from build123d import *

# Parameters (mm, degrees)
SKETCH1_W                  = 50
SKETCH1_H                  = 15
SKETCH1_R                  = 2.025
BASE_FLANGE1_DEPTH         = 1
F_4_CLEARANCE_HOLE1_D      = 3.2639
SKETCHED_START             = -7.5
SKETCHED_BEND1_DEPTH       = 15
SKETCHED_START_2           = -2.3680499
SKETCHED_BEND1_2_DEPTH     = 4.7360998
SKETCHED_BEND1_3_DEPTH     = 1.8680499
SKETCHED_START_3           = 5.6319501
SKETCHED_BEND1_4_DEPTH     = 1.8680499
SKETCHED_START_4           = -5.6319501
SKETCHED_BEND1_5_DEPTH     = 11.2639002
SKETCHED_START_5           = -15.8
SKETCHED_BEND1_6_OUTLINE_R = 1.63195
SKETCHED_BEND1_6_DEPTH     = 31.6
FILLET1_R                  = 2


with BuildPart() as part:
    # Base-Flange1: sheet metal written as solids
    # Sketch1 → Base-Flange1 (new body)
    with BuildSketch(Plane.XY):
        Rectangle(SKETCH1_W, SKETCH1_H)
        Circle(SKETCH1_R, mode=Mode.SUBTRACT)
    extrude(amount=-BASE_FLANGE1_DEPTH)

    # #4 Clearance Hole1 (through all)
    with Locations(Plane.XY):
        with Locations((-21, 4), (-21, -4), (21, 4), (21, -4)):
            Hole(F_4_CLEARANCE_HOLE1_D / 2)

    # Sketched Bend1: read off the stored shape, not the designer's step
    # Sketched Bend1 outline → Sketched Bend1 (cut)
    with BuildSketch(Plane(origin=(0, 0, 0), x_dir=(1, 0, 0), z_dir=(0, 1, 0)).offset(SKETCHED_START)):
        with BuildLine():
            ThreePointArc((-15.532050807, 0), (-14.8, 0.732050807), (-13.8, 1))
            Line((-13.8, 1), (-25, 1))
            Line((-25, 1), (-25, 0))
            Line((-25, 0), (-15.532050807, 0))
        make_face()
        with BuildLine():
            Line((25, 1), (13.8, 1))
            ThreePointArc((13.8, 1), (14.8, 0.732050807), (15.532050807, 0))
            Line((15.532050807, 0), (25, 0))
            Line((25, 0), (25, 1))
        make_face()
    extrude(amount=SKETCHED_BEND1_DEPTH, mode=Mode.SUBTRACT)

    # Sketched Bend1 2 outline → Sketched Bend1 2 (add)
    with BuildSketch(Plane(origin=(0, 0, 0), x_dir=(1, 0, 0), z_dir=(0, 1, 0)).offset(SKETCHED_START_2)):
        with BuildLine():
            Line((-13.8, 0), (-15.532050807, 0))
            ThreePointArc((-15.532050807, 0), (-15.731851652, -0.48236191), (-15.8, -1))
            Line((-15.8, -1), (-15.8, -9.84380551))
            Line((-15.8, -9.84380551), (-14.8, -9.84380551))
            Line((-14.8, -9.84380551), (-14.8, -1))
            ThreePointArc((-14.8, -1), (-14.507106781, -0.292893219), (-13.8, 0))
        make_face()
        with BuildLine():
            ThreePointArc((15.8, -1), (15.731851652, -0.48236191), (15.532050807, 0))
            Line((15.532050807, 0), (13.8, 0))
            ThreePointArc((13.8, 0), (14.507106781, -0.292893219), (14.8, -1))
            Line((14.8, -1), (14.8, -9.84380551))
            Line((14.8, -9.84380551), (15.8, -9.84380551))
            Line((15.8, -9.84380551), (15.8, -1))
        make_face()
    extrude(amount=SKETCHED_BEND1_2_DEPTH)

    # Sketched Bend1 3 outline → Sketched Bend1 3 (add)
    with BuildSketch(Plane(origin=(0, 0, 0), x_dir=(1, 0, 0), z_dir=(0, 1, 0)).offset(SKETCHED_START)):
        with BuildLine():
            Line((-13.8, 0), (-15.532050807, 0))
            ThreePointArc((-15.532050807, 0), (-15.731851652, -0.48236191), (-15.8, -1))
            Line((-15.8, -1), (-15.8, -9.84380551))
            Line((-15.8, -9.84380551), (-14.8, -9.84380551))
            Line((-14.8, -9.84380551), (-14.8, -1))
            ThreePointArc((-14.8, -1), (-14.507106781, -0.292893219), (-13.8, 0))
        make_face()
        with BuildLine():
            ThreePointArc((15.8, -1), (15.731851652, -0.48236191), (15.532050807, 0))
            Line((15.532050807, 0), (13.8, 0))
            ThreePointArc((13.8, 0), (14.507106781, -0.292893219), (14.8, -1))
            Line((14.8, -1), (14.8, -9.84380551))
            Line((14.8, -9.84380551), (15.8, -9.84380551))
            Line((15.8, -9.84380551), (15.8, -1))
        make_face()
    extrude(amount=SKETCHED_BEND1_3_DEPTH)

    # Sketched Bend1 4 outline → Sketched Bend1 4 (add)
    with BuildSketch(Plane(origin=(0, 0, 0), x_dir=(1, 0, 0), z_dir=(0, 1, 0)).offset(SKETCHED_START_3)):
        with BuildLine():
            Line((-13.8, 0), (-15.532050807, 0))
            ThreePointArc((-15.532050807, 0), (-15.731851652, -0.48236191), (-15.8, -1))
            Line((-15.8, -1), (-15.8, -9.84380551))
            Line((-15.8, -9.84380551), (-14.8, -9.84380551))
            Line((-14.8, -9.84380551), (-14.8, -1))
            ThreePointArc((-14.8, -1), (-14.507106781, -0.292893219), (-13.8, 0))
        make_face()
        with BuildLine():
            ThreePointArc((15.8, -1), (15.731851652, -0.48236191), (15.532050807, 0))
            Line((15.532050807, 0), (13.8, 0))
            ThreePointArc((13.8, 0), (14.507106781, -0.292893219), (14.8, -1))
            Line((14.8, -1), (14.8, -9.84380551))
            Line((14.8, -9.84380551), (15.8, -9.84380551))
            Line((15.8, -9.84380551), (15.8, -1))
        make_face()
    extrude(amount=SKETCHED_BEND1_4_DEPTH)

    # Sketched Bend1 5 outline → Sketched Bend1 5 (add)
    with BuildSketch(Plane(origin=(0, 0, 0), x_dir=(1, 0, 0), z_dir=(0, 1, 0)).offset(SKETCHED_START_4)):
        with BuildLine():
            Line((-13.8, 0), (-15.532050807, 0))
            ThreePointArc((-15.532050807, 0), (-15.731851652, -0.48236191), (-15.8, -1))
            Line((-15.8, -1), (-15.8, -9.84380551))
            Line((-15.8, -9.84380551), (-14.8, -9.84380551))
            Line((-14.8, -9.84380551), (-14.8, -1))
            ThreePointArc((-14.8, -1), (-14.507106781, -0.292893219), (-13.8, 0))
        make_face()
        with BuildLine():
            Line((15.532050807, 0), (13.8, 0))
            ThreePointArc((13.8, 0), (14.507106781, -0.292893219), (14.8, -1))
            Line((14.8, -1), (14.8, -9.84380551))
            Line((14.8, -9.84380551), (15.8, -9.84380551))
            Line((15.8, -9.84380551), (15.8, -1))
            ThreePointArc((15.8, -1), (15.731851652, -0.48236191), (15.532050807, 0))
        make_face()
    extrude(amount=SKETCHED_BEND1_5_DEPTH)

    # Sketched Bend1 6 outline → Sketched Bend1 6 (cut)
    with BuildSketch(Plane.YZ.offset(SKETCHED_START_5)):
        with Locations((-4, 5.84380551)):
            Circle(SKETCHED_BEND1_6_OUTLINE_R)
        with Locations((4, 5.84380551)):
            Circle(SKETCHED_BEND1_6_OUTLINE_R)
    extrude(amount=SKETCHED_BEND1_6_DEPTH, mode=Mode.SUBTRACT)

    # Fillet1
    fillet1_edges = [part.edges().sort_by_distance(p)[0] for p in [
        (15.3, 7.5, 9.84380551),
        (15.3, -7.5, 9.84380551),
        (-15.3, -7.5, 9.84380551),
        (-15.3, 7.5, 9.84380551),
    ]]
    fillet(fillet1_edges, radius=FILLET1_R)


solid = part.part
Model file for the job. Use its own axes, mm. A direction names the side the tool comes from. Round coordinates to 2 decimals unless told otherwise and drop trailing zeros. Order: outer loops, then holes, each group sorted by start corner. A loop starts at its lowest first (then second) coordinate and runs counter-clockwise, first axis right, second up. Notation, with made-up numbers: M -15,26 L 32,26 A19 cw 32,42 Z; hole C 79.5,18 d5. An arc over 180 degrees is marked long. Write each question's results on one line, items separated by ' | '. Start each with the question number.
(1) Saw through at A-A, the plane y = 4. Give the cut face in (x, z), then the cut area to 3 significant figures.
(2) Saw through at B-B, the plane x = 0. Give the cut face in (y, z) (3 decimals), then the cut area to 4 significant figures.
(3) Saw through at C-C, the plane y = 0. Give the cut face in (x, z) (3 decimals), then the cut area to 4 significant figures.
(4) Which spindle directions (+Z, -Z, +X, -X, +Y, -Y) get a long thin tool onto all of the face, cutting with end or side? Do faces 1 (the face through (14.499, -0.105, 0.285)), 2 (the face through (15.3, -2.5, 5.2)). Say none if no direction does.
(5) Two-plate mould, pull along Y, no slides. Class faces 3 (the face through (15.31, -6.93, 9.24)), 4 (the face through (15.31, 6.93, 9.24)), 5 (the face through (14.8, 0, 5)), 6 (the face through (15.293, 2.705, 4.851)): pulls with the +Y half, pulls with the -Y half, needs draft (parallel to the pull), parting line crosses it, or undercut.
(6) Probe probe 1 along X at (y, z) = (2.25, 2.25); probe 2 along Y at (x, z) = (0, -0.8) (3 decimals); probe 3 along Z at (x, y) = (-7, -5.5). List the from-to ranges inside material, lowest first. Write a range as from..to.
(7) Saw through at D-D, the plane z = 5.5. Give the cut face in (x, y), then the cut area to 3 significant figures.
(8) Drop flat-ended pins along their axis: pin 1 (4.5 mm diameter, centred on x = -4.5, y = -1, fed in from +Z); pin 2 (2.5 mm diameter, centred on y = 4, z = 5.84, fed in from +X). Give the stop position or say it passes through.
Established:
1) outline: M -15.8,1 A2 ccw -13.8,-1 L 13.8,-1 A2 ccw 15.8,1 L 15.8,4.21 L 14.8,4.21 L 14.8,1 A1 cw 13.8,0 L -13.8,0 A1 cw -14.8,1 L -14.8,4.21 L -15.8,4.21 Z; M -15.8,7.48 L -14.8,7.48 L -14.8,9.84 L -15.8,9.84 Z; M 14.8,7.48 L 15.8,7.48 L 15.8,9.84 L 14.8,9.84 Z | area: 43.5 mm^2
2) outline: M -7.5,-1 L -2.025,-1 L -2.025,0 L -7.5,0 Z; M 2.025,-1 L 7.5,-1 L 7.5,0 L 2.025,0 Z | area: 10.95 mm^2
3) outline: M -15.8,1 A2 ccw -13.8,-1 L -2.025,-1 L -2.025,0 L -13.8,0 A1 cw -14.8,1 L -14.8,9.844 L -15.8,9.844 Z; M 2.025,-1 L 13.8,-1 A2 ccw 15.8,1 L 15.8,9.844 L 14.8,9.844 L 14.8,1 A1 cw 13.8,0 L 2.025,0 Z | area: 45.95 mm^2
4) face 1: +Z, +Y, -Y | face 2: +X, -X
5) face 3: pulls with the -Y half | face 4: pulls with the +Y half | face 5: needs draft | face 6: undercut
6) probe 1: x = -15.8..-14.8, 14.8..15.8 | probe 2: y = -7.5..-2.025, 2.025..7.5 | probe 3: z = -1..0
7) outline: M -15.8,-7.5 L -14.8,-7.5 L -14.8,-5.6 L -15.8,-5.6 Z; M -15.8,-2.4 L -14.8,-2.4 L -14.8,2.4 L -15.8,2.4 Z; M -15.8,5.6 L -14.8,5.6 L -14.8,7.5 L -15.8,7.5 Z; M 14.8,-7.5 L 15.8,-7.5 L 15.8,-5.6 L 14.8,-5.6 Z; M 14.8,-2.4 L 15.8,-2.4 L 15.8,2.4 L 14.8,2.4 Z; M 14.8,5.6 L 15.8,5.6 L 15.8,7.5 L 14.8,7.5 Z | area: 17.2 mm^2
8) pin 1: stops at z = 0 | pin 2: passes through
